The model under review builds one solid part; all positions refer to its coordinate system, in mm. A direction names the side the tool comes from. Coordinates: 2 decimals unless noted, no trailing zeros. Order: outer loops, then holes, each group sorted by start corner. A loop starts at its lowest first (then second) coordinate and runs counter-clockwise, first axis right, second up. Notation, with made-up numbers: M 85.25,85.25 L 99.25,85.25 A16 ccw 99.25,92.25 Z; hole C 16,81.5 d7. An arc over 180 degrees is marked long. Answer as CSV lines item,"result". Start each with the question number.
Q1. Consider section B-B on x = 0. Write out the cut boundary in (y, z) (3 decimals).
Q2. Consider section D-D on z = 21. Write out the cut boundary in (x, y).
Q3. Consider section C-C on y = 23. Write out the cut boundary in (x, z).
Q4. The part is to be moulded in two halves that separate along Z. For faces 1 (the face through (47.333, -1.085, 14.906)), 2 (the face through (-39.626, -1.085, 0.049)), 3 (the face through (-22, 0, 30)), say which applies: +Z half, -Z half, draft (parallel to the pull), parting line (faces both ways), or undercut.
Q5. Wall thickness on L1, parallel to Z at x = 0, y = -1.5 (3 decimals); L2, parallel to Y at x = 3, z = -40; L3, parallel to X at y = 4.5, z = 4: over which ranges is each line inside the solid? List them lowest first. Write a range as [from, to].
Q6. For P1, Ø2, axis at x = 19.5, z = 7.5, coming from the -Y side; P2, Ø1.8, axis at x = 43.5, y = -1.5, coming from the -Z side; P3, Ø1.8, axis at x = -43, y = -0.5, coming from the -Z side, all flat-tipped, find the tip position at first contact; note any pin that passes through.
Q7. Consider section A-A on z = 0. Write out the cut boundary in (x, y) (3 decimals).
Q8. Machinability: for faces 4 (the face through (-34, -2.2, -10)), 5 (the face through (-46.624, -1.085, -0.049)), 6 (the face through (-28, -1, -21)), which of the approach directions +Z, -Z, +X, -X, +Y, -Y give a long, thin tool a straight path to every point of the face, cutting with its end or side? Answer none if there is none.
from build123d import *

# Parameters (mm, degrees)
F0_R     = 49.625
F0_R_2   = 35
F1_DEPTH = 2.2
F4_T     = 2.5


# Not quite as in the source:
# - a shell that OpenCascade refuses in one call is made with other operations: the cavity is built on its own and cut out
# - a feature names something its author has since deleted; it is built from what else it names


with BuildPart() as f1:
    # F0 (on Front) → F1 (new body)
    with BuildSketch(Plane.XZ):
        Circle(F0_R)
        with BuildLine():
            ThreePointArc((-44.375, -2.25), (-46.625, 0), (-44.375, 2.25))
            Line((-44.375, 2.25), (-41.875, 2.25))
            ThreePointArc((-41.875, 2.25), (-39.625, 0), (-41.875, -2.25))
            Line((-41.875, -2.25), (-44.375, -2.25))
        make_face(mode=Mode.SUBTRACT)
        Circle(F0_R_2, mode=Mode.SUBTRACT)
        with BuildLine():
            Line((44.375, -2.25), (41.875, -2.25))
            ThreePointArc((41.875, -2.25), (39.625, 0), (41.875, 2.25))
            Line((41.875, 2.25), (44.375, 2.25))
            ThreePointArc((44.375, 2.25), (46.625, 0), (44.375, -2.25))
        make_face(mode=Mode.SUBTRACT)
    extrude(amount=F1_DEPTH)

    # F2 (on Top) → F3 (revolve)
    with BuildSketch(Plane.XY):
        with BuildLine():
            Line((0, 0), (37, 0))
            ThreePointArc((37, 0), (26.1629509039, 26.1629509039), (0, 37))
            Line((0, 37), (0, 0))
        make_face()
    revolve(axis=Axis((0, 18.5, 0), (0, 1, 0)))

    # F4: shell of thickness 2.5, made by hand


with BuildPart() as f4_core1:
    # F4_t2: copy of F1
    add(f1.part)

    # the walls: a layer under each face that stays
    f4_faces = [f4_core1.faces().sort_by_distance(p)[0] for p in [
        (-49.625, -1.1, 0),
        (-33.0833333333, 0, -33.0833333333),
        (-33.0833333333, -2.2, -33.0833333333),
        (-46.625, -1.1, 0),
        (-43.125, -1.1, -2.25),
        (-43.125, -1.1, 2.25),
        (-39.625, -1.1, 0),
        (-26.1629509039, 26.1629509039, 0),
        (43.125, -1.1, -2.25),
        (46.625, -1.1, 0),
        (39.625, -1.1, 0),
        (43.125, -1.1, 2.25),
        (-35, -1.1, 0),
    ]]
    thicken(f4_faces, amount=-F4_T, mode=Mode.SUBTRACT)

    # F4_s3 → F4_t4 (revolve, cut)
    with BuildSketch(Plane.XY):
        Polygon((37.025, 0.025), (37, -2.5), (34.5, -2.5), (34.5, 0), align=None)
    revolve(axis=Axis((0, 0, 0), (0, 1, 0)), mode=Mode.SUBTRACT)


with BuildPart() as f1_1:
    add(f1.part)

    # what is left inside the walls is the cavity
    f4_cavity = [f4_core1.part.solids().sort_by_distance(p)[0] for p in [
        (-29.856226, 17.2375, 0),
    ]]
    add(f4_cavity, mode=Mode.SUBTRACT)


solid = f1_1.part
Evaluation:
1,outline,"M -2.2,-49.625 L 0,-49.625 L 0,-37 A37 ccw 0,37 L 0,49.625 L -2.2,49.625 L -2.2,35 L 0,35 L 0,34.5 A34.5 cw 0,-34.5 L 0,-35 L -2.2,-35 Z"
2,outline,"M -44.96,-2.2 L -28,-2.2 L -28,0 L -27.37,0 A27.37 cw 27.37,0 L 28,0 L 28,-2.2 L 44.96,-2.2 L 44.96,0 L 30.46,0 A30.46 ccw -30.46,0 L -44.96,0 Z"
3,outline,"C 0,0 d57.97; hole C 0,0 d51.43"
4,face 1,"parting line"
4,face 2,"undercut"
4,face 3,"draft"
5,L1,"z = [-49.625, -35], [35, 49.625]"
5,L2,"y = [-2.2, 0]"
5,L3,"x = [-36.51, -33.97], [33.97, 36.51]"
6,P1,"stops at y = 26.66"
6,P2,"stops at z = -25.45"
6,P3,"stops at z = -26.27"
7,outline,"M -49.625,-2.2 L -46.625,-2.2 L -46.625,0 L -49.625,0 Z; M -39.625,-2.2 L -35,-2.2 L -35,0 L -34.5,0 A34.5 cw 34.5,0 L 35,0 L 35,-2.2 L 39.625,-2.2 L 39.625,0 L 37,0 A37 ccw -37,0 L -39.625,0 Z; M 46.625,-2.2 L 49.625,-2.2 L 49.625,0 L 46.625,0 Z"
8,face 4,"+Z, -Z, +X, -X, -Y"
8,face 5,"+Y, -Y"
8,face 6,"-Y"
